Geometry check sheet. Reference: the model listing, model coordinates, mm. Face numbers are marked on the shaded views. A direction names the side the tool comes from. Give positions to 0.01 mm unless a question says otherwise; leave off trailing zeros. Loops run counter-clockwise (first coordinate to the right, second up) from the corner with the lowest first, then second, coordinate; pieces in that order, holes last. Notation, with made-up numbers: (-34, 88) -> (10, 88) arc R18 cw to (10, 104) -> close; hole circle Ø11 at (59.5, -1.75). An arc over 180 degrees is marked (long way). One line per item, written item: value. Start each with the question number.
(1) Sectioned sample at C-C, the plane x = 0. State how many separate pieces and enclosed holes the cut face has, then the cut area to 3 significant figures.
(2) Sectioned sample at A-A, the plane x = 70. Record the cut outline in (y, z).
(3) Scan lines: line 1 along X through (y, z) = (5.25, 0); line 2 along X through (y, z) = (4.75, 4.5); line 3 along X through (y, z) = (15.9, 0). Record each from-to range of solid material in increasing order. Write a range as from..to.
(4) Sectioned sample at B-B, the plane z = -70. Record the cut outline in (x, y).
(5) Tool access check on the marked faces 1, 2, 3, 4 and 5. Record the directions out of +Z, -Z, +X, -X, +Y, -Y that give a thin tool (end or side, any length) a straight path to the whole face; none if there is none.
(6) Gauge pin test, flat ends, axial feed: pin 1 Ø6.5 at (x, z) = (70, 0) entering from +Y; pin 2 Ø3 at (x, z) = (-19.5, 1.5) entering from -Y; pin 3 Ø2 at (x, y) = (-55, 17) entering from +Z; pin 4 Ø3 at (x, z) = (13, 13) entering from -Y. Record the tip position at first contact, or that the pin passes through.
from build123d import *

# Parameters (mm, degrees)
SKETCH1_W                               = 20
SKETCH1_H                               = 20
BOSS_EXTRUDE1_DEPTH                     = 20
CBORE_FOR_M5_HEX_HEAD_BOLT1_D           = 5.5
CBORE_FOR_M5_HEX_HEAD_BOLT1_CBORE_D     = 10.5
CBORE_FOR_M5_HEX_HEAD_BOLT1_CBORE_DEPTH = 10
CBORE_FOR_M5_HEX_HEAD_BOLT3_D           = 5.5
CBORE_FOR_M5_HEX_HEAD_BOLT3_CBORE_D     = 10.5
CBORE_FOR_M5_HEX_HEAD_BOLT3_CBORE_DEPTH = 14


with BuildPart() as part:
    # Sketch1 → Boss-Extrude1 (new body)
    with BuildSketch(Plane(origin=(0, 0, 0), x_dir=(1, 0, 0), z_dir=(0, 1, 0))):
        with BuildLine():
            ThreePointArc((-59.160797831, -10), (-60, 0), (-59.160797831, 10))
            Line((-59.160797831, 10), (-77.5, 10))
            ThreePointArc((-77.5, 10), (-79.267766953, 9.267766953), (-80, 7.5))
            Line((-80, 7.5), (-80, -7.5))
            ThreePointArc((-80, -7.5), (-79.267766953, -9.267766953), (-77.5, -10))
            Line((-77.5, -10), (-59.160797831, -10))
        make_face()
        with BuildLine():
            Line((-10, 10), (-10, 59.160797831))
            ThreePointArc((-10, 59.160797831), (-42.426406871, 42.426406871), (-59.160797831, 10))
            Line((-59.160797831, 10), (-10, 10))
        make_face()
        with BuildLine():
            Line((7.5, 80), (-7.5, 80))
            ThreePointArc((-7.5, 80), (-9.267766953, 79.267766953), (-10, 77.5))
            Line((-10, 77.5), (-10, 59.160797831))
            ThreePointArc((-10, 59.160797831), (0, 60), (10, 59.160797831))
            Line((10, 59.160797831), (10, 77.5))
            ThreePointArc((10, 77.5), (9.267766953, 79.267766953), (7.5, 80))
        make_face()
        with BuildLine():
            ThreePointArc((10, 59.160797831), (0, 60), (-10, 59.160797831))
            Line((-10, 59.160797831), (-10, 10))
            Line((-10, 10), (10, 10))
            Line((10, 10), (10, 59.160797831))
        make_face()
        with BuildLine():
            ThreePointArc((59.160797831, 10), (42.426406871, 42.426406871), (10, 59.160797831))
            Line((10, 59.160797831), (10, 10))
            Line((10, 10), (59.160797831, 10))
        make_face()
        with BuildLine():
            Line((77.5, 10), (59.160797831, 10))
            ThreePointArc((59.160797831, 10), (59.789831367, 5.017575617), (60, 0))
            ThreePointArc((60, 0), (59.789831367, -5.017575617), (59.160797831, -10))
            Line((59.160797831, -10), (77.5, -10))
            ThreePointArc((77.5, -10), (79.267766953, -9.267766953), (80, -7.5))
            Line((80, -7.5), (80, 7.5))
            ThreePointArc((80, 7.5), (79.267766953, 9.267766953), (77.5, 10))
        make_face()
        with BuildLine():
            Line((59.160797831, 10), (10, 10))
            Line((10, 10), (10, -10))
            Line((10, -10), (59.160797831, -10))
            ThreePointArc((59.160797831, -10), (59.789831367, -5.017575617), (60, 0))
            ThreePointArc((60, 0), (59.789831367, 5.017575617), (59.160797831, 10))
        make_face()
        Rectangle(SKETCH1_W, SKETCH1_H)
        with BuildLine():
            Line((-10, -10), (-10, 10))
            Line((-10, 10), (-59.160797831, 10))
            ThreePointArc((-59.160797831, 10), (-60, 0), (-59.160797831, -10))
            Line((-59.160797831, -10), (-10, -10))
        make_face()
        with BuildLine():
            Line((-10, -59.160797831), (-10, -10))
            Line((-10, -10), (-59.160797831, -10))
            ThreePointArc((-59.160797831, -10), (-42.426406871, -42.426406871), (-10, -59.160797831))
        make_face()
        with BuildLine():
            Line((59.160797831, -10), (10, -10))
            Line((10, -10), (10, -59.160797831))
            ThreePointArc((10, -59.160797831), (42.426406871, -42.426406871), (59.160797831, -10))
        make_face()
        with BuildLine():
            Line((10, -10), (-10, -10))
            Line((-10, -10), (-10, -59.160797831))
            ThreePointArc((-10, -59.160797831), (0, -60), (10, -59.160797831))
            Line((10, -59.160797831), (10, -10))
        make_face()
        with BuildLine():
            ThreePointArc((10, -59.160797831), (0, -60), (-10, -59.160797831))
            Line((-10, -59.160797831), (-10, -77.5))
            ThreePointArc((-10, -77.5), (-9.267766953, -79.267766953), (-7.5, -80))
            Line((-7.5, -80), (7.5, -80))
            ThreePointArc((7.5, -80), (9.267766953, -79.267766953), (10, -77.5))
            Line((10, -77.5), (10, -59.160797831))
        make_face()
    extrude(amount=BOSS_EXTRUDE1_DEPTH)

    # CBORE for M5 Hex Head Bolt1 (through all)
    with Locations(Plane(origin=(0, 20, -70), x_dir=(0, 0, 1), z_dir=(0, 1, 0))):
        with Locations((0, 0), (70, 70), (70, -70), (140, 0)):
            CounterBoreHole(CBORE_FOR_M5_HEX_HEAD_BOLT1_D / 2, CBORE_FOR_M5_HEX_HEAD_BOLT1_CBORE_D / 2, CBORE_FOR_M5_HEX_HEAD_BOLT1_CBORE_DEPTH)

    # CBORE for M5 Hex Head Bolt3 (through all)
    with Locations(Plane(origin=(0, 0, -18), x_dir=(0, 0, -1), z_dir=(0, -1, 0))):
        with Locations((0, 0), (-5.272077939, -12.727922061), (-18, -18), (-30.727922061, -12.727922061), (-36, 0), (-30.727922061, 12.727922061), (-18, 18), (-5.272077939, 12.727922061)):
            CounterBoreHole(CBORE_FOR_M5_HEX_HEAD_BOLT3_D / 2, CBORE_FOR_M5_HEX_HEAD_BOLT3_CBORE_D / 2, CBORE_FOR_M5_HEX_HEAD_BOLT3_CBORE_DEPTH)


solid = part.part
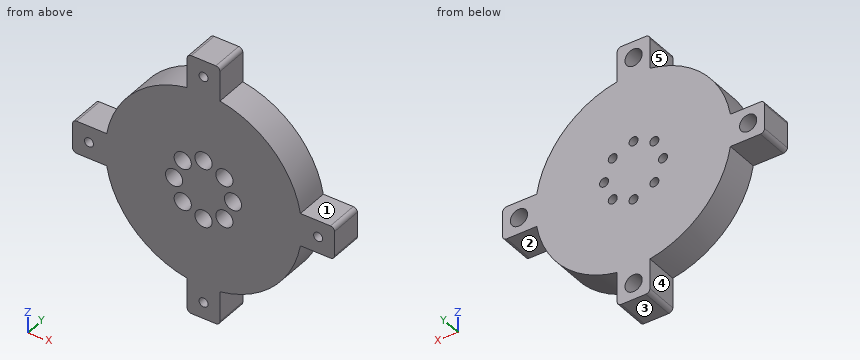
Calculated:
1. separate pieces: 5
1. enclosed holes: 0
1. area: 2,520 mm2
2. outline: (0, -10) -> (20, -10) -> (20, -5.25) -> (10, -5.25) -> (10, -2.75) -> (0, -2.75) -> close; (0, 2.75) -> (10, 2.75) -> (10, 5.25) -> (20, 5.25) -> (20, 10) -> (0, 10) -> close
3. line 1: x = -80..-72.75, -67.25..-23.25, -12.75..12.75, 23.25..67.25, 72.75..80
3. line 2: x = -80..-20.7, -15.3..15.3, 20.7..80
3. line 3: x = -80..-75.25, -64.75..-20.75, -15.25..15.25, 20.75..64.75, 75.25..80
4. outline: (-10, 0) -> (-2.75, 0) -> (-2.75, 10) -> (-5.25, 10) -> (-5.25, 20) -> (-10, 20) -> close; (2.75, 0) -> (10, 0) -> (10, 20) -> (5.25, 20) -> (5.25, 10) -> (2.75, 10) -> close
5. face 1: +Z, +X, +Y, -Y
5. face 2: -Z, +X, +Y, -Y
5. face 3: -Z, +X, -X, +Y, -Y
5. face 4: -Z, -X, +Y, -Y
5. face 5: +Z, -X, +Y, -Y
6. pin 1: stops at y = 10
6. pin 2: stops at y = 14
6. pin 3: stops at z = 26.15
6. pin 4: passes through
